Check sheet for the modelled part. Datum: model origin and axes. Units: mm. A direction names the side the tool comes from. Give positions to 0.01 mm unless a question says otherwise; leave off trailing zeros. Write each loop counter-clockwise with the first axis right and the second up, starting at its lowest first coordinate (ties: lowest second). Pieces come first, ordered by that corner, then holes. Notation, with made-up numbers: (85.25, -12.5) -> (122.25, -12.5) arc R16 cw to (122.25, 15.5) -> close; hole circle Ø10 at (-27, 38.5). An arc over 180 degrees is marked (long way). Answer as a JSON object with one key per item and string values.
from build123d import *

# Parameters (mm, degrees)
SKETCH_R   = 10.75
SKETCH_R_2 = 1.75
SKETCH_W   = 45.6
SKETCH_H   = 27
PAD_DEPTH  = 3.5


with BuildPart() as part:
    # Sketch → Pad (new body)
    with BuildSketch(Plane.XY):
        with BuildLine():
            Line((-67, 50), (67, 50))
            ThreePointArc((70, 47), (69.12132, 49.12132), (67, 50))
            Line((70, 47), (70, -47))
            ThreePointArc((67, -50), (69.12132, -49.12132), (70, -47))
            Line((67, -50), (-67, -50))
            ThreePointArc((-70, -47), (-69.12132, -49.12132), (-67, -50))
            Line((-70, -47), (-70, 47))
            ThreePointArc((-67, 50), (-69.12132, 49.12132), (-70, 47))
        make_face()
        with Locations((-42, -24)):
            Circle(SKETCH_R, mode=Mode.SUBTRACT)
        with Locations((42, -24)):
            Circle(SKETCH_R, mode=Mode.SUBTRACT)
        with Locations((-60, 40)):
            Circle(SKETCH_R_2, mode=Mode.SUBTRACT)
        with Locations((60, 40)):
            Circle(SKETCH_R_2, mode=Mode.SUBTRACT)
        with Locations((-60, -40)):
            Circle(SKETCH_R_2, mode=Mode.SUBTRACT)
        with Locations((60, -40)):
            Circle(SKETCH_R_2, mode=Mode.SUBTRACT)
        with Locations((0, -24)):
            Circle(SKETCH_R, mode=Mode.SUBTRACT)
        with Locations((-31.8, 23.5)):
            Rectangle(SKETCH_W, SKETCH_H, mode=Mode.SUBTRACT)
        with Locations((31.8, 23.5)):
            Rectangle(SKETCH_W, SKETCH_H, mode=Mode.SUBTRACT)
    extrude(amount=PAD_DEPTH)


solid = part.part
1. Go/stop test with flat-tipped pins: P1, Ø19.5, axis at x = 42, y = -24, coming from the -Z side; P2, Ø10, axis at x = 47, y = 4, coming from the -Z side. Record where each tip stops, or that it passes through.
Determined:
{"P1": "through", "P2": "z = 0"}
2. Scan lines: L1, parallel to X at y = 16.5, z = 3.3; L2, parallel to Y at x = 60, z = 2.75; L3, parallel to Y at x = 0, z = 1.6. Record each from-to range of solid material in increasing order. Write a range as [from, to].
Determined:
{"L1": "[-70, -54.6], [-9, 9], [54.6, 70]", "L2": "[-50, -41.75], [-38.25, 38.25], [41.75, 50]", "L3": "[-50, -34.75], [-13.25, 50]"}
3. Mould release check, pull along X, two halves, no side actions. Record for faces 1 (the face through (70, 1, 2)), 2 (the face through (-54.6, 23, 2)), 3 (the face through (-1, 50, 2)): released by +X, released by -X, zero draft, split by the parting line, or undercut.
Determined:
{"face 1": "released by +X", "face 2": "undercut", "face 3": "zero draft"}
4. Access from +Z, -Z, +X, -X, +Y, -Y to the whole of each face (thin tool, end or side, straight path). Record for faces 4 (the face through (1, 1, 3.5)), 5 (the face through (9, 23, 2)).
Determined:
{"face 4": "+Z, +X, -X, +Y, -Y", "face 5": "+Z, -Z"}
5. Sectioned sample at B-B, the plane z = 2.2. State how many separate pieces and enclosed holes the cut face has, plus the area to 3 significant figures.
Determined:
{"separate pieces": "1", "enclosed holes": "9", "area": "10,400 mm^2"}
6. Sectioned sample at D-D, the plane x = 0. Enter the section's corners in (y, z).
Determined:
{"outline": "(-50, 0) -> (-34.75, 0) -> (-34.75, 3.5) -> (-50, 3.5) -> close; (-13.25, 0) -> (50, 0) -> (50, 3.5) -> (-13.25, 3.5) -> close"}
7. Sectioned sample at C-C, the plane x = -60. Enter the section's corners in (y, z).
Determined:
{"outline": "(-50, 0) -> (-41.75, 0) -> (-41.75, 3.5) -> (-50, 3.5) -> close; (-38.25, 0) -> (38.25, 0) -> (38.25, 3.5) -> (-38.25, 3.5) -> close; (41.75, 0) -> (50, 0) -> (50, 3.5) -> (41.75, 3.5) -> close"}
8. Sectioned sample at A-A, the plane y = -24. Enter the section's corners in (x, z), plus the area to 3 significant figures.
Determined:
{"outline": "(-70, 0) -> (-52.75, 0) -> (-52.75, 3.5) -> (-70, 3.5) -> close; (-31.25, 0) -> (-10.75, 0) -> (-10.75, 3.5) -> (-31.25, 3.5) -> close; (10.75, 0) -> (31.25, 0) -> (31.25, 3.5) -> (10.75, 3.5) -> close; (52.75, 0) -> (70, 0) -> (70, 3.5) -> (52.75, 3.5) -> close", "area": "264 mm^2"}
